```python
from build123d import *

# Parameters (mm, degrees)
F0_W     = 50.8
F0_H     = 25.4
F0_W_2   = 44.45
F0_H_2   = 19.05
F1_DEPTH = 254
F2_R     = 3.2385
F2_R_2   = 6.35
F2_R_3   = 2.5781
F3_DEPTH = 25.4
F4_R     = 2.5781
F5_DEPTH = 50.801
F7_DEPTH = 50.801


with BuildPart() as f1:
    # F0 (on Front) → F1 (new body)
    with BuildSketch(Plane.XZ):
        with Locations((-25.4, 12.7)):
            Rectangle(F0_W, F0_H)
        with Locations((-25.4, 12.7)):
            Rectangle(F0_W_2, F0_H_2, mode=Mode.SUBTRACT)
    extrude(amount=F1_DEPTH)

    # F2 (on face) → F3 (cut)
    with BuildSketch(Plane.XY.offset(25.4)):
        with Locations((-25.4, -63.5)):
            Circle(F2_R)
        with Locations((-25.4, -25.4)):
            Circle(F2_R)
        with Locations((-25.4, -107.95)):
            Circle(F2_R_2)
        with Locations((-44.45, -133.35)):
            Circle(F2_R_3)
        with Locations((-38.1, -133.35)):
            Circle(F2_R_3)
        with Locations((-12.7, -133.35)):
            Circle(F2_R_3)
        with Locations((-6.35, -133.35)):
            Circle(F2_R_3)
        with Locations((-44.45, -193.675)):
            Circle(F2_R_3)
        with Locations((-38.1, -193.675)):
            Circle(F2_R_3)
        with Locations((-12.7, -193.675)):
            Circle(F2_R_3)
        with Locations((-6.35, -193.675)):
            Circle(F2_R_3)
    extrude(amount=-F3_DEPTH, mode=Mode.SUBTRACT)

    # F4 (on face) → F5 (cut, through all)
    with BuildSketch(Plane.YZ):
        with Locations((-241.3, 12.7)):
            Circle(F4_R)
        with Locations((-215.9, 12.7)):
            Circle(F4_R)
    extrude(amount=-F5_DEPTH, mode=Mode.SUBTRACT)

    # F6 (on face) → F7 (cut, through all)
    with BuildSketch(Plane(origin=(-50.8, 0, 0), x_dir=(0, -1, 0), z_dir=(-1, 0, 0))):
        with BuildLine():
            Line((201.66838, 22.225), (185.68162, 22.225))
            ThreePointArc((185.68162, 22.225), (184.598601, 21.776399), (184.15, 20.69338))
            Line((184.15, 20.69338), (184.15, 4.70662))
            ThreePointArc((184.15, 4.70662), (184.598601, 3.623601), (185.68162, 3.175))
            Line((185.68162, 3.175), (201.66838, 3.175))
            ThreePointArc((201.66838, 3.175), (202.751399, 3.623601), (203.2, 4.70662))
            Line((203.2, 4.70662), (203.2, 20.69338))
            ThreePointArc((203.2, 20.69338), (202.751399, 21.776399), (201.66838, 22.225))
        make_face()
        with BuildLine():
            Line((141.34338, 22.225), (125.35662, 22.225))
            ThreePointArc((125.35662, 22.225), (124.273601, 21.776399), (123.825, 20.69338))
            Line((123.825, 20.69338), (123.825, 4.70662))
            ThreePointArc((123.825, 4.70662), (124.273601, 3.623601), (125.35662, 3.175))
            Line((125.35662, 3.175), (141.34338, 3.175))
            ThreePointArc((141.34338, 3.175), (142.426399, 3.623601), (142.875, 4.70662))
            Line((142.875, 4.70662), (142.875, 20.69338))
            ThreePointArc((142.875, 20.69338), (142.426399, 21.776399), (141.34338, 22.225))
        make_face()
    extrude(amount=-F7_DEPTH, mode=Mode.SUBTRACT)


solid = f1.part
```
Geometry: final body of the model. Coordinates: model frame, mm. A direction names the side the tool comes from. Coordinates: 2 decimals unless noted, no trailing zeros. Loops run counter-clockwise (first coordinate to the right, second up) from the corner with the lowest first, then second, coordinate; pieces in that order, holes last. Notation, with made-up numbers: (35.25, -7) -> (70.25, -7) arc R13 ccw to (70.25, 3) -> close; hole circle Ø11 at (73, 8.25). An arc over 180 degrees is marked (long way). Use a Markdown table: item, result. Add a question column.
(1) Access query for faces 1 (the cylindrical face through (-35.64, -132.58, 1.61)), 2 (the flat face through (-3.175, -163, 13)). Directions: +Z, -Z, +X, -X, +Y, -Y. A direction counts if a zero-diameter tool reaches every point of the face in a straight line with its end or side. Return the directions, or none.
(2) Line query: line 1 along Y through (x, z) = (-6.35, 23.9); line 2 along X through (y, z) = (-133.35, 2.3); line 3 along Z through (x, y) = (-27.5, -214) (3 decimals). Output: solid intervals per line, ascending.
(3) Section query C-C, the plane x = -25.4. State how many separate pieces and enclosed holes the cut face has, plus the area to 3 significant figures.
(4) Section query A-A, the plane y = -215.9. Return loops of the section in (x, z) (3 decimals).
(5) Section query B-B, the plane x = -12.7. Return loops of the section in (y, z) (3 decimals).
(6) Mould query, pull axis X, two halves, no side actions, for faces 3 (the flat face through (0, -125, 24)), 4 (the cylindrical face through (-27.787, -23.211, 1.61)), 5 (the cylindrical face through (-1.57, -213.44, 13.47)). Classes: pulls with the +X half, pulls with the -X half, needs draft (parallel to the pull), parting line crosses it, or undercut.
(7) Pin query (flat end, axial travel): pin 1 Ø4.5 at (x, y) = (-6.35, -193.675) entering from +Z. Return the tip coordinate at first contact, or that it passes through.
Answer:
| question | item | result |
|---|---|---|
| 1 | face 1 | +Z, -Z |
| 1 | face 2 | +Y, -Y |
| 2 | line 1 | y = -254 to -196.25, -191.1 to -135.93, -130.77 to 0 |
| 2 | line 2 | x = -50.8 to -47.03, -41.87 to -40.68, -35.52 to -15.28, -10.12 to -8.93, -3.77 to 0 |
| 2 | line 3 | z = 0 to 3.175, 22.225 to 25.4 |
| 3 | separate pieces | 8 |
| 3 | enclosed holes | 0 |
| 3 | area | 1,450 mm^2 |
| 4 | outline | (-50.8, 0) -> (0, 0) -> (0, 10.122) -> (-3.175, 10.122) -> (-3.175, 3.175) -> (-47.625, 3.175) -> (-47.625, 10.122) -> (-50.8, 10.122) -> close; (-50.8, 15.278) -> (-47.625, 15.278) -> (-47.625, 22.225) -> (-3.175, 22.225) -> (-3.175, 15.278) -> (0, 15.278) -> (0, 25.4) -> (-50.8, 25.4) -> close |
| 5 | outline | (-254, 0) -> (-196.253, 0) -> (-196.253, 3.175) -> (-254, 3.175) -> close; (-254, 22.225) -> (-196.253, 22.225) -> (-196.253, 25.4) -> (-254, 25.4) -> close; (-191.097, 0) -> (-135.928, 0) -> (-135.928, 3.175) -> (-191.097, 3.175) -> close; (-191.097, 22.225) -> (-135.928, 22.225) -> (-135.928, 25.4) -> (-191.097, 25.4) -> close; (-130.772, 0) -> (0, 0) -> (0, 3.175) -> (-130.772, 3.175) -> close; (-130.772, 22.225) -> (0, 22.225) -> (0, 25.4) -> (-130.772, 25.4) -> close |
| 6 | face 3 | pulls with the +X half |
| 6 | face 4 | undercut |
| 6 | face 5 | needs draft |
| 7 | pin 1 | passes through |
